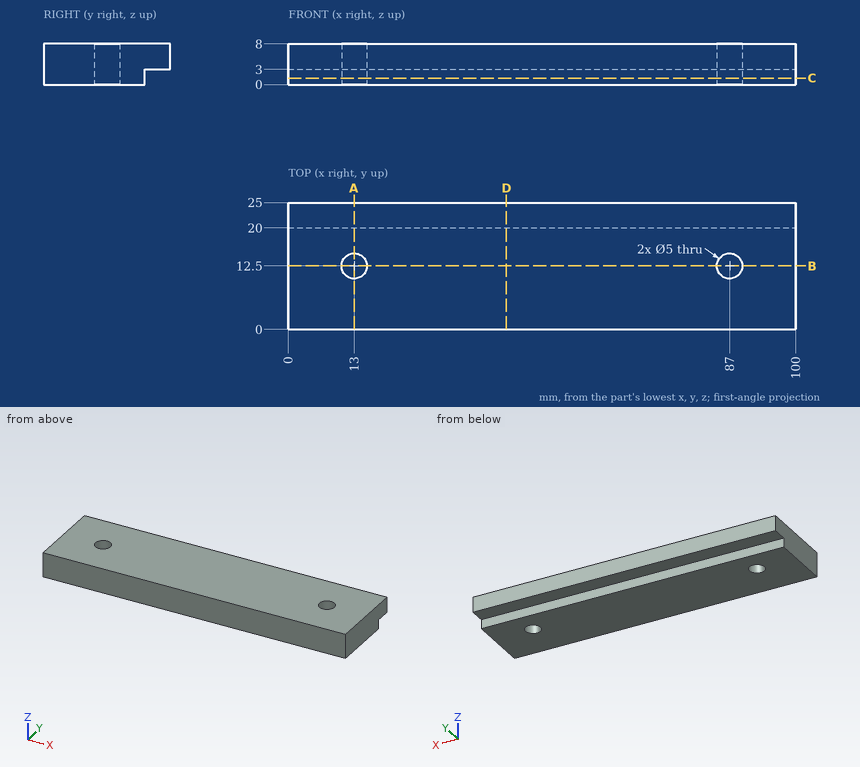
Verification items for this drawing (mm, ordinates from the low corner). Give positions to 0.01 mm unless a question says otherwise; leave off trailing zeros. Loops run counter-clockwise (first coordinate to the right, second up) from the corner with the lowest first, then second, coordinate; pieces in that order, holes last. Notation, with made-up numbers: M 61.25,79.5 L 71.25,79.5 A21 ccw 71.25,116.5 Z; hole C 36.5,-34.5 d4. An arc over 180 degrees is marked long. Answer as a JSON object with one key per item and string values. Group by question number.
Q1. Cross-section at D-D on x = 43. Record the cut outline in (y, z), then the cut area to 3 significant figures.
Q2. Cross-section at B-B on y = 12.5. Record the cut outline in (x, z).
Q3. Go/stop test with flat-tipped pins: P1, Ø1.5, axis at x = 28, y = 21.5, coming from the -Z side; P2, Ø2.5, axis at x = 29.5, z = 1, coming from the +Y side. Record where each tip stops, or that it passes through.
Q4. Cross-section at A-A on x = 13. Record the cut outline in (y, z), then the cut area to 3 significant figures.
Q5. Material ranges on line 1 along Y through (x, z) = (13, 3.75); line 2 along Y through (x, z) = (87, 2.5); line 3 along Y through (x, z) = (48, 1.5), recorded low to high. Write a range as [from, to].
Q6. Cross-section at C-C on z = 1.25. Record the cut outline in (x, y).
Evaluation:
{
 "1": {"outline": "M 0,0 L 20,0 L 20,3 L 25,3 L 25,8 L 0,8 Z", "area": "185 mm2"},
 "2": {"outline": "M 0,0 L 10.5,0 L 10.5,8 L 0,8 Z; M 15.5,0 L 84.5,0 L 84.5,8 L 15.5,8 Z; M 89.5,0 L 100,0 L 100,8 L 89.5,8 Z"},
 "3": {"P1": "stops at z = 3", "P2": "stops at y = 20"},
 "4": {"outline": "M 0,0 L 10,0 L 10,8 L 0,8 Z; M 15,0 L 20,0 L 20,3 L 25,3 L 25,8 L 15,8 Z", "area": "145 mm2"},
 "5": {"line 1": "y = [0, 10], [15, 25]", "line 2": "y = [0, 10], [15, 20]", "line 3": "y = [0, 20]"},
 "6": {"outline": "M 0,0 L 100,0 L 100,20 L 0,20 Z; hole C 13,12.5 d5; hole C 87,12.5 d5"}
}
